```python
from build123d import *

# Parameters (mm, degrees)
F0_W      = 105
F0_H      = 35
F1_DEPTH  = 7
F2_W      = 70
F2_H      = 19
F3_DEPTH  = 7.001
F5_DEPTH  = 7.001
F7_DEPTH  = 7.001
F8_W      = 65
F8_H      = 5
F9_DEPTH  = 7.001
F10_W     = 65
F10_H     = 5
F11_DEPTH = 7.001
F12_W     = 5
F12_H     = 35
F13_DEPTH = 5
F14_W     = 12
F14_H     = 35
F15_DEPTH = 7
F16_R     = 2
F17_DEPTH = 1
F18_R     = 0.5


with BuildPart() as f1:
    # F0 (on Top) → F1 (new body)
    with BuildSketch(Plane.XY):
        Rectangle(F0_W, F0_H)
    extrude(amount=F1_DEPTH)

    # F2 (on face) → F3 (cut, through all)
    with BuildSketch(Plane.XY.offset(7)):
        with Locations((17.5, 0)):
            Rectangle(F2_W, F2_H)
    extrude(amount=-F3_DEPTH, mode=Mode.SUBTRACT)

    # F4 (on face) → F5 (cut, through all)
    with BuildSketch(Plane.XY.offset(7)):
        Polygon((52.5, 17.5), (47.5, 17.5), (52.5, 9.5), align=None)
    extrude(amount=-F5_DEPTH, mode=Mode.SUBTRACT)

    # F6 (on face) → F7 (cut, through all)
    with BuildSketch(Plane.XY.offset(7)):
        Polygon((52.5, -9.5), (47.5, -17.5), (52.5, -17.5), align=None)
    extrude(amount=-F7_DEPTH, mode=Mode.SUBTRACT)

    # F8 (on face) → F9 (cut, through all)
    with BuildSketch(Plane.XY.offset(7)):
        with Locations((15, 15)):
            Rectangle(F8_W, F8_H)
    extrude(amount=-F9_DEPTH, mode=Mode.SUBTRACT)

    # F10 (on face) → F11 (cut, through all)
    with BuildSketch(Plane.XY.offset(7)):
        with Locations((15, -15)):
            Rectangle(F10_W, F10_H)
    extrude(amount=-F11_DEPTH, mode=Mode.SUBTRACT)

    # F12 (on face) → F13 (join)
    with BuildSketch(Plane.XY.offset(7)):
        with Locations((-20, 0)):
            Rectangle(F12_W, F12_H)
    extrude(amount=F13_DEPTH)

    # F14 (on face) → F15 (join)
    with BuildSketch(Plane.XY.offset(7)):
        with Locations((-46.5, 0)):
            Rectangle(F14_W, F14_H)
    extrude(amount=F15_DEPTH)

    # F16
    f16_edges = [f1.edges().sort_by_distance(p)[0] for p in [
        (-40.5, 0, 14),
        (-46.5, 17.5, 14),
        (-46.5, -17.5, 14),
        (-52.5, 0, 14),
    ]]
    fillet(f16_edges, radius=F16_R)

    # F17 (cut): faces of the model
    f17_faces = [f1.faces().sort_by_distance(p)[0] for p in [
        (18.1782945736, -11.1085271318, 7),
        (18.1782945736, 11.1085271318, 7),
    ]]
    extrude(f17_faces, amount=-F17_DEPTH, mode=Mode.SUBTRACT)

    # F18
    f18_edges = [f1.edges().sort_by_distance(p)[0] for p in [
        (-17.5, -12.5, 3),
        (-17.5, -11, 6),
        (-17.5, 9.5, 3),
        (-17.5, 11, 6),
        (-17.5, -9.5, 3),
        (-17.5, 12.5, 3),
    ]]
    fillet(f18_edges, radius=F18_R)


solid = f1.part
```
Check sheet for the modelled part. Datum: model origin and axes. Units: mm. A direction names the side the tool comes from. Give positions to 0.01 mm unless a question says otherwise; leave off trailing zeros. Write each loop counter-clockwise with the first axis right and the second up, starting at its lowest first coordinate (ties: lowest second). Pieces come first, ordered by that corner, then holes.
Item 1: Gauge pin test, flat ends, axial feed: pin 1 (3 mm diameter, centred on x = 0.5, z = 3.5, fed in from +Y); pin 2 (9 mm diameter, centred on x = -34, y = 0.5, fed in from +Z); pin 3 (4 mm diameter, centred on x = 31, y = -12.5, fed in from +Z); pin 4 (12 mm diameter, centred on x = -7, y = 2.5, fed in from -Z). Record the tip position at first contact, or that the pin passes through.
Item 2: Scan lines: L1, parallel to Y at x = 27.5, z = 5; L2, parallel to X at y = -14, z = 8.25; L3, parallel to Z at x = -37, y = 0.5. Record each from-to range of solid material in increasing order.
Item 3: Cross-section at C-C (y = -14). Enter the section's corners in (x, z), and give its area (3 significant figures).
Item 4: Cross-section at B-B (x = 33). Enter the section's corners in (y, z).
Item 5: Cross-section at D-D (z = 4.25). Enter the section's corners in (x, y), and give its area (3 significant figures).
Item 6: Draft check along Y on faces 1 (the face through (-22.5, 0, 9)), 2 (the face through (15, -12.5, 3)), 3 (the face through (49.965, 13.556, 3.042)), 4 (the face through (-17.5, 0, 6)). Enter one of: released by +Y, released by -Y, zero draft, split by the parting line, or undercut.
Item 7: Cross-section at A-A (z = 10.5). Enter the section's corners in (x, y).
Item 8: Access from +Z, -Z, +X, -X, +Y, -Y to the whole of each face (thin tool, end or side, straight path). Record for faces 5 (the face through (25, -12, 6)), 6 (the face through (17, -9.5, 3)), 7 (the face through (15, 12.5, 3)), 8 (the face through (-40.5, 0, 9)).
Report:
1. pin 1: stops at y = 12.5
1. pin 2: stops at z = 7
1. pin 3: stops at z = 6
1. pin 4: passes through
2. L1: y = -12.5 to -9.5, 9.5 to 12.5
2. L2: x = -52.5 to -40.5, -22.5 to -17.5
2. L3: z = 0 to 7
3. outline: (-52.5, 0) - (-17.5, 0) - (-17.5, 12) - (-22.5, 12) - (-22.5, 7) - (-40.5, 7) - (-40.5, 12) arc R2 ccw to (-42.5, 14) - (-50.5, 14) arc R2 ccw to (-52.5, 12) - close; (47.5, 0) - (49.69, 0) - (49.69, 6) - (47.5, 6) - close
3. area: 365 mm2
4. outline: (-12.5, 0) - (-9.5, 0) - (-9.5, 6) - (-12.5, 6) - close; (9.5, 0) - (12.5, 0) - (12.5, 6) - (9.5, 6) - close
5. outline: (-52.5, -17.5) - (-17.5, -17.5) - (-17.5, -13) arc R0.5 cw to (-17, -12.5) - (47.5, -12.5) - (47.5, -17.5) - (52.5, -9.5) - (-17, -9.5) arc R0.5 cw to (-17.5, -9) - (-17.5, 9) arc R0.5 cw to (-17, 9.5) - (52.5, 9.5) - (47.5, 17.5) - (47.5, 12.5) - (-17, 12.5) arc R0.5 cw to (-17.5, 13) - (-17.5, 17.5) - (-52.5, 17.5) - close
5. area: 1,660 mm2
6. face 1: zero draft
6. face 2: released by -Y
6. face 3: released by +Y
6. face 4: undercut
7. outline: (-52.5, -17.5) - (-40.5, -17.5) - (-40.5, 17.5) - (-52.5, 17.5) - close; (-22.5, -17.5) - (-17.5, -17.5) - (-17.5, 17.5) - (-22.5, 17.5) - close
8. face 5: +Z, +X, +Y, -Y
8. face 6: +Z, -Z, +X
8. face 7: +Z, -Z, +Y
8. face 8: +Z, +Y, -Y
